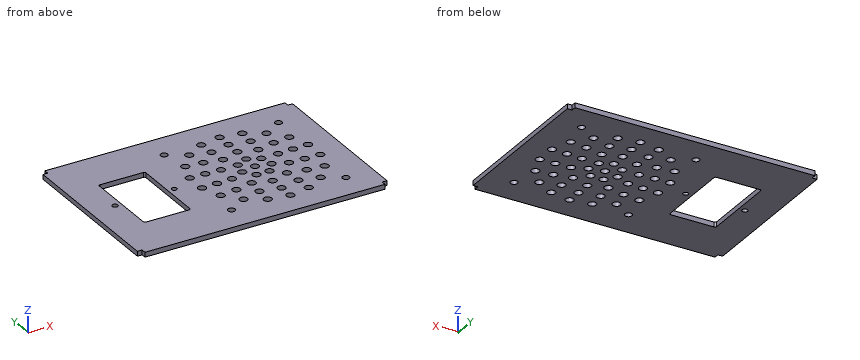
Autodesk Fusion 360 part; units mm, degrees
sketch "Esquisse1" plane through (0, 0, 0) normal (0, 0, 1) x (1, 0, 0)
  line L0 (75, -53) -> (-75, -53)
  line L1 (-75, -53) -> (-75, 53)
  line L2 (-75, 53) -> (75, 53)
  line L3 (75, 53) -> (75, -53)
  line L4 (75, -53) -> (-75, 53) construction
  line L5 (-75, -53) -> (75, 53) construction
  line L6 (78, 50) -> (-78, 50)
  line L7 (-78, 50) -> (-78, -50)
  line L8 (-78, -50) -> (78, -50)
  line L9 (78, -50) -> (78, 50)
  line L10 (78, 50) -> (-78, -50) construction
  line L11 (-78, 50) -> (78, -50) construction
  dimension "d1" = 150
  dimension "d2" = 106
  dimension "d49" = 156
  dimension "d50" = 100
extrude "Extrusion1" add sketch "Esquisse1" along normal blind 3
sketch "Esquisse4" plane through (0, 0, 3) normal (0, 0, 1) x (-1, 0, 0)
  line L0 (-75, -53) -> (75, -53)
  line L1 (75, -53) -> (75, -50)
  line L2 (75, 53) -> (-75, 53)
  line L3 (-75, -50) -> (-75, -53)
  circle A0 centre (-25, -37.5) radius 2.5
  circle A1 centre (-25, -28.125) radius 2.5
  circle A2 centre (-25, -18.75) radius 2.5
  circle A3 centre (-25, -9.375) radius 2.5
  circle A4 centre (-25, 0) radius 2.5
  circle A5 centre (-12.1742, -35.2385) radius 2.5
  circle A6 centre (-0.8955, -28.7267) radius 2.5
  circle A7 centre (7.476, -18.75) radius 2.5
  circle A8 centre (11.9303, -6.5118) radius 2.5
  circle A9 centre (11.9303, 6.5118) radius 2.5
  circle A10 centre (7.476, 18.75) radius 2.5
  circle A11 centre (-0.8955, 28.7267) radius 2.5
  circle A12 centre (-12.1742, 35.2385) radius 2.5
  circle A13 centre (-25, 37.5) radius 2.5
  circle A14 centre (-37.8258, 35.2385) radius 2.5
  circle A15 centre (-49.1045, 28.7267) radius 2.5
  circle A16 centre (-57.476, 18.75) radius 2.5
  circle A17 centre (-61.9303, 6.5118) radius 2.5
  circle A18 centre (-61.9303, -6.5118) radius 2.5
  circle A19 centre (-57.476, -18.75) radius 2.5
  circle A20 centre (-49.1045, -28.7267) radius 2.5
  circle A21 centre (-37.8258, -35.2385) radius 2.5
  circle A22 centre (-12.797, -25.3397) radius 2.5
  circle A23 centre (-3.011, -17.5357) radius 2.5
  circle A24 centre (2.4198, -6.2584) radius 2.5
  circle A25 centre (2.4198, 6.2584) radius 2.5
  circle A26 centre (-3.011, 17.5357) radius 2.5
  circle A27 centre (-12.797, 25.3397) radius 2.5
  circle A28 centre (-25, 28.125) radius 2.5
  circle A29 centre (-37.203, 25.3397) radius 2.5
  circle A30 centre (-46.989, 17.5357) radius 2.5
  circle A31 centre (-52.4198, 6.2584) radius 2.5
  circle A32 centre (-52.4198, -6.2584) radius 2.5
  circle A33 centre (-46.989, -17.5357) radius 2.5
  circle A34 centre (-37.203, -25.3397) radius 2.5
  circle A35 centre (-13.979, -15.1691) radius 2.5
  circle A36 centre (-7.1677, -5.7941) radius 2.5
  circle A37 centre (-7.1677, 5.7941) radius 2.5
  circle A38 centre (-13.979, 15.1691) radius 2.5
  circle A39 centre (-25, 18.75) radius 2.5
  circle A40 centre (-36.021, 15.1691) radius 2.5
  circle A41 centre (-42.8323, 5.7941) radius 2.5
  circle A42 centre (-42.8323, -5.7941) radius 2.5
  circle A43 centre (-36.021, -15.1691) radius 2.5
  circle A44 centre (-17.6703, -5.8452) radius 2.5
  circle A45 centre (-15.8601, 2.0861) radius 2.5
  circle A46 centre (-20.9323, 8.4466) radius 2.5
  circle A47 centre (-29.0677, 8.4466) radius 2.5
  circle A48 centre (-34.1399, 2.0861) radius 2.5
  circle A49 centre (-32.3297, -5.8452) radius 2.5
  line L4 (-75, 50) -> (-78, 50)
  line L5 (-78, 50) -> (-78, -50)
  line L6 (-78, -50) -> (-75, -50)
  line L7 (75, -50) -> (78, -50)
  line L8 (78, -50) -> (78, 50)
  line L9 (78, 50) -> (75, 50)
  line L10 (75, 50) -> (75, 53)
  line L11 (-75, 53) -> (-75, 50)
  circle A50 centre (-60.75, -35.75) radius 2.2
  circle A51 centre (10.75, 35.75) radius 2.2
  line L12 (-60.75, -35.75) -> (10.75, -35.75)
  line L13 (10.75, 35.75) -> (-60.75, -35.75) construction
  line L14 (-60.75, 35.75) -> (10.75, -35.75) construction
  circle A52 centre (10.75, -35.75) radius 2.2
  line L15 (10.75, 35.75) -> (-60.75, 35.75)
  line L16 (-60.75, 35.75) -> (-60.75, -35.75)
  line L17 (10.75, -35.75) -> (10.75, 35.75)
  circle A53 centre (-60.75, 35.75) radius 2.2
  line L18 (-75, 50) -> (-78, 50)
  point P0 (-25, 0)
  dimension "d32" = 5
  dimension "d37" = 0
  dimension "d38" = 37.5
  dimension "d40" = 360
  dimension "d42" = 360
  dimension "d44" = 360
  dimension "d46" = 360
  dimension "d51" = 71.5
  dimension "d52" = 71.5
  dimension "d53" = 4.4
  dimension "d54" = 4.4
  dimension "d55" = 4.4
  dimension "d56" = 4.4
extrude "Extrusion5" cut sketch "Esquisse4" against normal blind 3 contours A0 L12 | A0 L12 | A5 L12 | A5 L12 | A21 L12 | A21 L12 | L12 A52 L17 | L12 A52 L17 | A50 L12 L16 | A50 L12 L16 | A8 L17 | A8 L17 | A18 L16 | A18 L16 | A9 L17 | A9 L17 | A17 L16 | A17 L16 | A51 L15 L17 | A51 L15 L17 | L15 L16 A53 | L15 L16 A53 | A12 L15 | A12 L15 | A14 L15 | A14 L15 | A13 L15 | A13 L15 | A1 | A2 | A3 | A4 | A6 | A7 | A10 | A11 | A15 | A16 | A19 | A20 | A22 | A23 | A24 | A25 | A26 | A27 | A28 | A29 | A30 | A31 | A32 | A33 | A34 | A35 | A36 | A37 | A38 | A39 | A40 | A41 | A42 | A43 | A44 | A45 | A46 | A47 | A48 | A49
sketch "Esquisse3" plane through (0, 0, 0) normal (0, 0, 1) x (1, 0, 0)
  line L0 (-29.3032, 23.4839) -> (-29.3032, -23.1161)
  line L1 (-29.3032, -24.1161) -> (-58.4032, 24.4839) construction
  line L2 (-58.4032, -23.1161) -> (-58.4032, 23.4839)
  line L3 (-57.4032, 24.4839) -> (-30.3032, 24.4839)
  line L4 (-58.4032, -24.1161) -> (-29.3032, 24.4839) construction
  circle A0 centre (-25.3532, 0.1839) radius 1.625
  circle A1 centre (-62.3532, 0.1839) radius 1.75
  circle A2 centre (-25.3532, 0.1839) radius 1.75 construction
  arc A3 (-58.4032, -23.1161) -> (-57.4032, -24.1161) centre (-57.4032, -23.1161) ccw
  arc A4 (-29.3032, 23.4839) -> (-30.3032, 24.4839) centre (-30.3032, 23.4839) ccw
  arc A5 (-30.3032, -24.1161) -> (-29.3032, -23.1161) centre (-30.3032, -23.1161) ccw
  arc A6 (-57.4032, 24.4839) -> (-58.4032, 23.4839) centre (-57.4032, 23.4839) ccw
  line L5 (-30.3032, -24.1161) -> (-57.4032, -24.1161)
  dimension "d26" = 1
  dimension "d27" = 3.5
  dimension "d28" = 3.5
extrude "Extrusion4" cut sketch "Esquisse3" along normal blind 3
Here's how the part is built. I have some questions about the finished solid (model axes, mm). Round coordinates to 2 decimals unless told otherwise and drop trailing zeros. Write each loop counter-clockwise with the first axis right and the second up, starting at its lowest first coordinate (ties: lowest second). Pieces come first, ordered by that corner, then holes.
Q1. If we section it at A-A on x = -55: Write out the boundary of the cut face in (y, z), plus the area to 3 significant figures.
Q2. If we section it at B-B on z = 1.55: Give the number of separate pieces and of enclosed holes in the cut face, plus the area to 3 significant figures.
Q3. Will this pin go through, and if not, where does the flat tip stop? P1, Ø6.5, axis at x = 12.17, y = -35.24, coming from the -Z side.
Q4. Please list where these lines run through material, in increasing order: probe 1 along Y at (x, z) = (7, 2.45); probe 2 along X at (y, z) = (-25, 1.6); probe 3 along X at (y, z) = (-11.5, 2.8).
Answer below:
1. outline: (-53, 0) - (-24.12, 0) - (-24.12, 3) - (-53, 3) - close; (24.48, 0) - (53, 0) - (53, 3) - (24.48, 3) - close
1. area: 172 mm2
2. separate pieces: 1
2. enclosed holes: 57
2. area: 14,000 mm2
3. P1: stops at z = 0
4. probe 1: y = -53 to -8.29, -3.3 to 3.3, 8.29 to 53
4. probe 2: x = -78 to 10.32, 15.27 to 34.73, 39.68 to 78
4. probe 3: x = -78 to -58.4, -29.3 to 78
